```python
from build123d import *

# Parameters (mm, degrees)
SKETCH1_R           = 9.398
SKETCH1_R_2         = 1.4351
BOSS_EXTRUDE1_DEPTH = 5.715
SKETCH2_R           = 5.7404
BOSS_EXTRUDE2_DEPTH = 3.683


with BuildPart() as part:
    # Sketch1 → Boss-Extrude1 (new body)
    with BuildSketch(Plane.XY):
        Circle(SKETCH1_R)
        Circle(SKETCH1_R_2, mode=Mode.SUBTRACT)
    extrude(amount=BOSS_EXTRUDE1_DEPTH)

    # Sketch2 → Boss-Extrude2 (add)
    with BuildSketch(Plane(origin=(0, 0, 0), x_dir=(-1, 0, 0), z_dir=(0, 0, -1))):
        with Locations(Location((0, 0, 0), (0, 0, 180))):
            Circle(SKETCH2_R)
        Polygon((3.764397664, 3.359086542), (3.359739968, -3.752913458), (-3.752260032, -3.348255763), (-3.347602336, 3.763744237), align=None, mode=Mode.SUBTRACT)
    extrude(amount=BOSS_EXTRUDE2_DEPTH)


solid = part.part
```
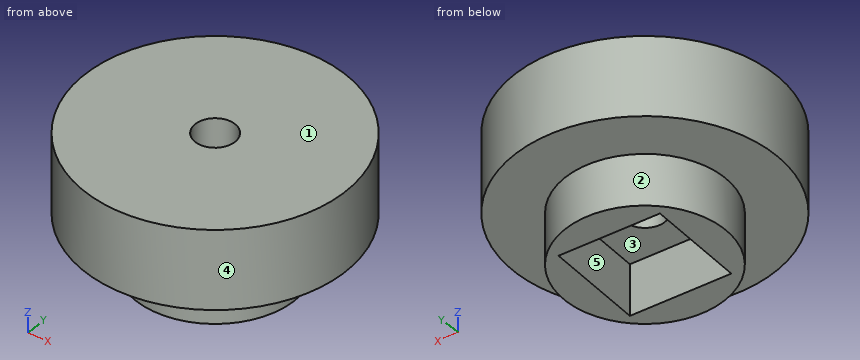
Model file for the job. Use its own axes, mm. Face numbers are marked on the shaded views. A direction names the side the tool comes from. Give positions to 0.01 mm unless a question says otherwise; leave off trailing zeros. Order: outer loops, then holes, each group sorted by start corner. A loop starts at its lowest first (then second) coordinate and runs counter-clockwise, first axis right, second up.
1) Saw through at C-C, the plane z = 1. Write the cut outline in (x, y), then the cut area to 3 significant figures.
2) Saw through at A-A, the plane y = 0.25. Write the cut outline in (x, z) (1 decimal).
3) Wall check: probe 1 along Y at (x, z) = (0, 4); probe 2 along Z at (x, y) = (4.25, 5.5) (3 decimals); probe 3 along X at (y, z) = (2.5, -2.25). Give the ranges that are in metal, low to high.
4) Mould opens along Y. For the marked faces 1, 2 and 3 say: +Y half, -Y half, draft (parallel to the pull), parting line (faces both ways), or undercut.
5) Pin check, flat tips, straight feed: pin 1 (2.5 mm diameter, centred on x = 0, y = 0, fed in from -Z); pin 2 (2.5 mm diameter, centred on x = 0, y = -1, fed in from -Z); pin 3 (3 mm diameter, centred on x = -2.5, z = -2.5, fed in from +Y). Stop position of each tip, or through.
6) Saw through at B-B, the plane x = 0. Write the cut outline in (y, z) (3 decimals), then the cut area to 3 significant figures.
7) 3-axis set-ups, long thin cutter, end or side, ignore diameter. For the marked faces 4 and 5: which of +Z, -Z, +X, -X, +Y, -Y reach the whole face in a straight line?
8) Saw through at D-D, the plane y = 2.75. Write the cut outline in (x, z) (3 decimals).
Computed:
1. outline: circle Ø18.8 at (0, 0); hole circle Ø2.87 at (0, 0)
1. area: 271 mm2
2. outline: (-9.4, 0) - (-5.7, 0) - (-5.7, -3.7) - (-3.6, -3.7) - (-3.6, 0) - (-1.4, 0) - (-1.4, 5.7) - (-9.4, 5.7) - close; (1.4, 0) - (3.5, 0) - (3.5, -3.7) - (5.7, -3.7) - (5.7, 0) - (9.4, 0) - (9.4, 5.7) - (1.4, 5.7) - close
3. probe 1: y = -9.4 to -1.44, 1.44 to 9.4
3. probe 2: z = 0 to 5.715
3. probe 3: x = -5.17 to -3.72, 3.42 to 5.17
4. face 1: draft
4. face 2: parting line
4. face 3: undercut
5. pin 1: passes through
5. pin 2: stops at z = 0
5. pin 3: stops at y = 5.65
6. outline: (-9.398, 0) - (-5.74, 0) - (-5.74, -3.683) - (-3.562, -3.683) - (-3.562, 0) - (-1.435, 0) - (-1.435, 5.715) - (-9.398, 5.715) - close; (1.435, 0) - (3.573, 0) - (3.573, -3.683) - (5.74, -3.683) - (5.74, 0) - (9.398, 0) - (9.398, 5.715) - (1.435, 5.715) - close
6. area: 107 mm2
7. face 4: +Z, -Z
7. face 5: -Z
8. outline: (-8.987, 0) - (-5.039, 0) - (-5.039, -3.683) - (-3.73, -3.683) - (-3.73, 0) - (3.405, 0) - (3.405, -3.683) - (5.039, -3.683) - (5.039, 0) - (8.987, 0) - (8.987, 5.715) - (-8.987, 5.715) - close
